```python
from build123d import *

# Parameters (mm, degrees)
BOSS_EXTRUDE1_DEPTH = 19.05


with BuildPart() as part:
    # Sketch1 → Boss-Extrude1 (new body)
    with BuildSketch(Plane(origin=(0, 0, 0), x_dir=(1, 0, 0), z_dir=(0, 1, 0))):
        Polygon((172.509838787, 0), (159.378309213, 66.016657224), (121.982876828, 121.982876828), (66.016657224, 159.378309213), (0, 172.509838787), (-66.016657224, 159.378309213), (-121.982876828, 121.982876828), (-159.378309213, 66.016657224), (-172.509838787, 0), (-159.378309213, -66.016657224), (-121.982876828, -121.982876828), (-66.016657224, -159.378309213), (0, -172.509838787), (66.016657224, -159.378309213), (121.982876828, -121.982876828), (159.378309213, -66.016657224), align=None)
        Polygon((129.778773347, 0), (119.89995245, 49.664186433), (91.767450688, 91.767450688), (49.664186433, 119.89995245), (0, 129.778773347), (-49.664186433, 119.89995245), (-91.767450688, 91.767450688), (-119.89995245, 49.664186433), (-129.778773347, 0), (-119.89995245, -49.664186433), (-91.767450688, -91.767450688), (-49.664186433, -119.89995245), (0, -129.778773347), (49.664186433, -119.89995245), (91.767450688, -91.767450688), (119.89995245, -49.664186433), align=None, mode=Mode.SUBTRACT)
    extrude(amount=BOSS_EXTRUDE1_DEPTH)


solid = part.part
```
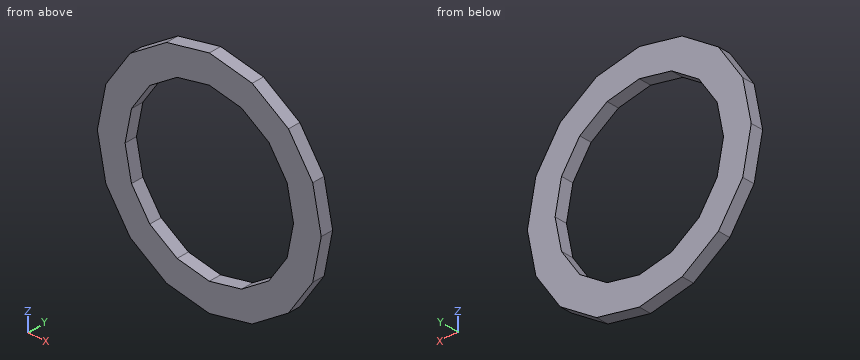
Verification items for the finished model (mm, model axes). Coordinates: 2 decimals unless noted, no trailing zeros. Loops run counter-clockwise (first coordinate to the right, second up) from the corner with the lowest first, then second, coordinate; pieces in that order, holes last. Notation, with made-up numbers: (79.25, 40.5) - (87.25, 40.5) arc R11 ccw to (87.25, 58.5) - close; hole circle Ø4 at (89, 2.25). An arc over 180 degrees is marked (long way). Return JSON: item names as keys, results as strings.
1. Section check C-C, the plane x = -25. Record the boundary of the cut face in (y, z).
Established:
{"outline": "(0, -167.54) - (19.05, -167.54) - (19.05, -124.81) - (0, -124.81) - close; (0, 124.81) - (19.05, 124.81) - (19.05, 167.54) - (0, 167.54) - close"}
2. Section check B-B, the plane z = 16.5. Record the boundary of the cut face in (x, y), then the cut area to 3 significant figures.
Established:
{"outline": "(-169.23, 0) - (-126.5, 0) - (-126.5, 19.05) - (-169.23, 19.05) - close; (126.5, 0) - (169.23, 0) - (169.23, 19.05) - (126.5, 19.05) - close", "area": "1,630 mm2"}
3. Go/stop test with flat-tipped pins: pin 1 (4 mm diameter, centred on y = 4, z = 3.5, fed in from -X); pin 2 (1.5 mm diameter, centred on x = -31, y = 9.5, fed in from +Z); pin 3 (1 mm diameter, centred on x = -84.5, y = 6, fed in from +Z). Record where each tip stops, or that it passes through.
Established:
{"pin 1": "stops at x = -172.21", "pin 2": "stops at z = 166.49", "pin 3": "stops at z = 147.36"}
4. Section check D-D, the plane z = -149. Record the boundary of the cut face in (x, y), then the cut area to 3 significant figures.
Established:
{"outline": "(-81.55, 0) - (81.55, 0) - (81.55, 19.05) - (-81.55, 19.05) - close", "area": "3,110 mm2"}
5. Thickness scan on L1, parallel to X at y = 13.25, z = 37.5; L2, parallel to X at y = 5.5, z = -71. Record the ranges inside material, lowest first.
Established:
{"L1": "x = -165.05 to -122.32, 122.32 to 165.05", "L2": "x = -156.05 to -105.64, 105.64 to 156.05"}
